Here's the drawing with two shaded views (mm, measured from the low corner). I have some questions. A direction names the side the tool comes from. Round coordinates to 2 decimals unless told otherwise and drop trailing zeros. Order: outer loops, then holes, each group sorted by start corner. A loop starts at its lowest first (then second) coordinate and runs counter-clockwise, first axis right, second up.
Q1. If we section it at B-B (x = 125): Please give me the cut outline in (y, z), plus the area to 4 significant figures.
Q2. We'd pull the mould along X, two halves only. Please class the marked faces 6, 7 and 8: pulls with the +X half, pulls with the -X half, needs draft (parallel to the pull), parting line crosses it, or undercut.
Q3. Will these pins go through, and if not, where does the flat tip stop? P1, Ø1, axis at y = 78.5, z = 42, coming from the -X side; P2, Ø1, axis at y = 51, z = 94, coming from the -X side.
Q4. If I drill on line 1 (Z direction, x = 125, y = 119.75); line 2 (Z direction, x = 75, y = 113); line 3 (Y direction, x = 43, z = 121), over which ranges is the centre line in solid material (lowest first)?
Q5. For the marked faces 1, 2, 3, 4 and 5, which set-ups out of +Z, -Z, +X, -X, +Y, -Y let a thin tool reach every point of the face, with its end or its side?
Q6. If we section it at A-A (z = 175): Please give me the cut outline in (x, y).
Q7. If we section it at D-D (z = 148): Please give me the cut outline in (x, y).
Q8. If we section it at C-C (y = 53): Please give me the cut outline in (x, z), plus the area to 3 significant figures.
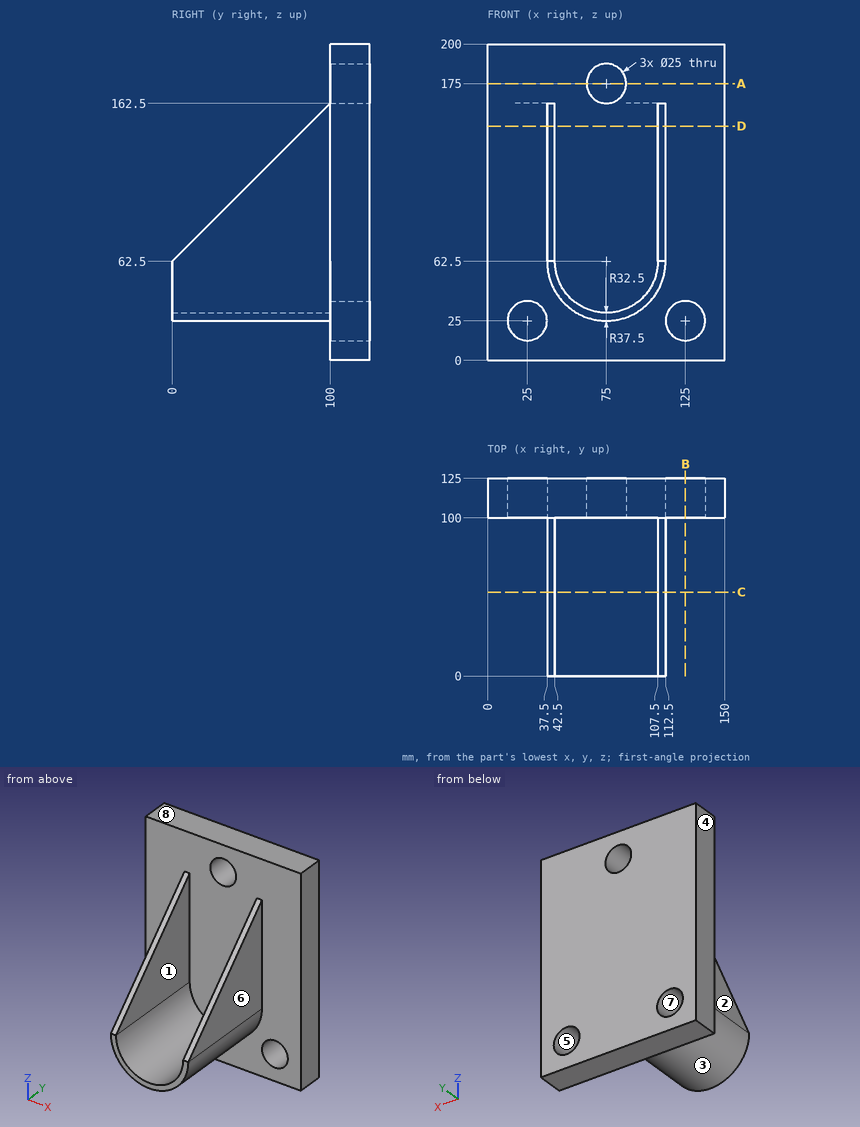
Solution:
1. outline: (100, 0) - (125, 0) - (125, 12.5) - (100, 12.5) - close; (100, 37.5) - (125, 37.5) - (125, 200) - (100, 200) - close
1. area: 4,375 mm2
2. face 6: pulls with the +X half
2. face 7: undercut
2. face 8: needs draft
3. P1: stops at x = 43.28
3. P2: stops at x = 37.5
4. line 1: z = 0 to 12.5, 37.5 to 200
4. line 2: z = 0 to 162.5, 187.5 to 200
4. line 3: y = 100 to 125
5. face 1: +Z, -Y
5. face 2: +Z, -Z, -X, -Y
5. face 3: -Z, -Y
5. face 4: +Z, -Z, -X, +Y, -Y
5. face 5: +Y, -Y
6. outline: (0, 100) - (62.5, 100) - (62.5, 125) - (0, 125) - close; (87.5, 100) - (150, 100) - (150, 125) - (87.5, 125) - close
7. outline: (0, 100) - (37.5, 100) - (37.5, 85.5) - (42.5, 85.5) - (42.5, 100) - (107.5, 100) - (107.5, 85.5) - (112.5, 85.5) - (112.5, 100) - (150, 100) - (150, 125) - (0, 125) - close
8. outline: (37.5, 62.5) arc R37.5 ccw to (112.5, 62.5) - (112.5, 115.5) - (107.5, 115.5) - (107.5, 62.5) arc R32.5 cw to (42.5, 62.5) - (42.5, 115.5) - (37.5, 115.5) - close
8. area: 1,080 mm2
